Geometry check sheet. Reference: the model listing, model coordinates, mm. A direction names the side the tool comes from. Round coordinates to 2 decimals unless told otherwise and drop trailing zeros. Write each loop counter-clockwise with the first axis right and the second up, starting at its lowest first coordinate (ties: lowest second). Pieces come first, ordered by that corner, then holes. Notation, with made-up numbers: (63.25, 1) -> (74.25, 1) arc R26 ccw to (74.25, 19) -> close; hole circle Ø10 at (5.25, 68). An arc over 180 degrees is marked (long way). Use a Markdown table: item, result.
```python
from build123d import *

# Parameters (mm, degrees)
F0_R      = 50
F1_DEPTH  = 1
F2_R      = 47.5
F3_DEPTH  = 4
F4_R      = 50
F4_R_2    = 47.5
F5_DEPTH  = 1
F7_DEPTH  = 6
F8_DEPTH  = 1
F9_R      = 5
F10_DEPTH = 25


with BuildPart() as f1:
    # F0 (on Front) → F1 (new body)
    with BuildSketch(Plane.XZ):
        Circle(F0_R)
    extrude(amount=F1_DEPTH)

    # F2 (on face) → F3 (join)
    with BuildSketch(Plane.XZ.offset(1)):
        Circle(F2_R)
    extrude(amount=F3_DEPTH)

    # F4 (on face) → F5 (join)
    with BuildSketch(Plane.XZ.offset(5)):
        Circle(F4_R)
        Circle(F4_R_2, mode=Mode.SUBTRACT)
    extrude(amount=F5_DEPTH)

    # F6 (on face) → F7 (join)
    with BuildSketch(Plane.XZ.offset(5)):
        with BuildLine():
            ThreePointArc((4.3749025625, 8.5724532519), (2.590430401, 7.6252153584), (1.4813797084, 9.3138855699))
            ThreePointArc((1.4813797084, 9.3138855699), (0.0968585728, 11.046369539), (-1.4993910756, 9.5067635707))
            ThreePointArc((-1.4993910756, 9.5067635707), (-2.3862869161, 7.6915455975), (-4.2761032204, 8.4058248554))
            ThreePointArc((-4.2761032204, 8.4058248554), (-6.4145328749, 8.9936327239), (-6.8009682853, 6.8098133285))
            ThreePointArc((-6.8009682853, 6.8098133285), (-6.4515237381, 4.8199668444), (-8.4002600583, 4.2870247495))
            ThreePointArc((-8.4002600583, 4.2870247495), (-10.4757907864, 3.5056338906), (-9.5048067664, 1.5117458519))
            ThreePointArc((-9.5048067664, 1.5117458519), (-8.0524977714, 0.1073245813), (-9.3158030683, -1.4692731))
            ThreePointArc((-9.3158030683, -1.4692731), (-10.5356526766, -3.3213979368), (-8.5781321192, -4.3637571578))
            ThreePointArc((-8.5781321192, -4.3637571578), (-6.5776913503, -4.6463120239), (-6.6730259387, -6.6643585641))
            ThreePointArc((-6.6730259387, -6.6643585641), (-6.5712533379, -8.8797686425), (-4.3749025625, -8.5724532519))
            ThreePointArc((-4.3749025625, -8.5724532519), (-2.590430401, -7.6252153584), (-1.4813797084, -9.3138855699))
            ThreePointArc((-1.4813797084, -9.3138855699), (-0.0968585728, -11.046369539), (1.4993910756, -9.5067635707))
            ThreePointArc((1.4993910756, -9.5067635707), (2.3862869161, -7.6915455975), (4.2761032204, -8.4058248554))
            ThreePointArc((4.2761032204, -8.4058248554), (6.4145328749, -8.9936327239), (6.8009682853, -6.8098133285))
            ThreePointArc((6.8009682853, -6.8098133285), (6.4515237381, -4.8199668444), (8.4002600583, -4.2870247495))
            ThreePointArc((8.4002600583, -4.2870247495), (10.4757907864, -3.5056338906), (9.5048067664, -1.5117458519))
            ThreePointArc((9.5048067664, -1.5117458519), (8.0524977714, -0.1073245813), (9.3158030683, 1.4692731))
            ThreePointArc((9.3158030683, 1.4692731), (10.5356526766, 3.3213979368), (8.5781321192, 4.3637571578))
            ThreePointArc((8.5781321192, 4.3637571578), (6.5776913503, 4.6463120239), (6.6730259387, 6.6643585641))
            ThreePointArc((6.6730259387, 6.6643585641), (6.5712533379, 8.8797686425), (4.3749025625, 8.5724532519))
        make_face()
    extrude(amount=F7_DEPTH)

    # F8 (add): a face of the model
    f8_faces = [f1.faces().sort_by_distance(p)[0] for p in [
        (-46.1564971157, -5, 0),
    ]]
    extrude(f8_faces, amount=F8_DEPTH)

    # F9 (on face) → F10 (cut)
    with BuildSketch(Plane.XZ.offset(11)):
        Circle(F9_R)
    extrude(amount=-F10_DEPTH, mode=Mode.SUBTRACT)


solid = f1.part
```
(1) Thickness scan on line 1 (Z direction, x = 0, y = -8); line 2 (Y direction, x = -42, z = 26); line 3 (Z direction, x = 0, y = -5.75). Record the ranges inside material, lowest first.
A:
| item | result |
|---|---|
| line 1 | z = -11.05 to -5, 5 to 11.05 |
| line 2 | y = -6 to -5, -1 to 0 |
| line 3 | z = -50 to -5, 5 to 50 |
(2) Section check A-A on x = 0. Record the cut outline in (y, z).
A:
| item | result |
|---|---|
| outline | (-11, -11.05) -> (-6, -11.05) -> (-6, -50) -> (-5, -50) -> (-5, -47.5) -> (-1, -47.5) -> (-1, -50) -> (0, -50) -> (0, -5) -> (-11, -5) -> close; (-11, 5) -> (0, 5) -> (0, 50) -> (-1, 50) -> (-1, 47.5) -> (-5, 47.5) -> (-5, 50) -> (-6, 50) -> (-6, 11.05) -> (-11, 11.05) -> close |
(3) Section check C-C on z = 38. Record the cut outline in (x, y).
A:
| item | result |
|---|---|
| outline | (-32.5, -6) -> (32.5, -6) -> (32.5, -5) -> (28.5, -5) -> (28.5, -1) -> (32.5, -1) -> (32.5, 0) -> (-32.5, 0) -> (-32.5, -1) -> (-28.5, -1) -> (-28.5, -5) -> (-32.5, -5) -> close |
(4) Gauge pin test, flat ends, axial feed: pin 1 Ø6 at (x, y) = (1.5, -3) entering from -Z; pin 2 Ø8 at (x, z) = (0, 0) entering from -Y; pin 3 Ø4 at (y, z) = (-1, -22.5) entering from -X; pin 4 Ø2 at (y, z) = (-2.5, 28.5) entering from +X. Record the tip position at first contact, or that the pin passes through.
A:
| item | result |
|---|---|
| pin 1 | stops at z = -50 |
| pin 2 | passes through |
| pin 3 | stops at x = -45.6 |
| pin 4 | stops at x = 38.73 |
(5) Section check B-B on z = 0. Record the cut outline in (x, y).
A:
| item | result |
|---|---|
| outline | (-50, -6) -> (-8.05, -6) -> (-8.05, -11) -> (-5, -11) -> (-5, 0) -> (-50, 0) -> (-50, -1) -> (-47.5, -1) -> (-47.5, -5) -> (-50, -5) -> close; (5, -11) -> (8.05, -11) -> (8.05, -6) -> (50, -6) -> (50, -5) -> (47.5, -5) -> (47.5, -1) -> (50, -1) -> (50, 0) -> (5, 0) -> close |
(6) Section check D-D on y = -3. Record the cut outline in (x, z).
A:
| item | result |
|---|---|
| outline | circle Ø95 at (0, 0); hole circle Ø10 at (0, 0) |
(7) Release check for a two-part mould opening along Z. For faces 4 (the face through (47.69, -0.49, 15.02)), 5 (the face through (5, -11, 3)), 6 (the face through (-1.08, -5.58, -4.88)) record: +Z half, -Z half, draft (parallel to the pull), parting line (faces both ways), or undercut.
A:
| item | result |
|---|---|
| face 4 | parting line |
| face 5 | draft |
| face 6 | undercut |
(8) Access from +Z, -Z, +X, -X, +Y, -Y to the whole of each face (thin tool, end or side, straight path). Record for faces 1 (the face through (47.69, -5.49, 15.02)), 2 (the face through (-10.3, -2.97, -46.37)), 3 (the face through (10, -6, 1)).
A:
| item | result |
|---|---|
| face 1 | +Y, -Y |
| face 2 | none |
| face 3 | -Y |
